Can you work these out from the model? Positions are in its coordinate system, mm. A direction names the side the tool comes from. Coordinates: 2 decimals unless noted, no trailing zeros. Loops run counter-clockwise (first coordinate to the right, second up) from the corner with the lowest first, then second, coordinate; pieces in that order, holes last.
Autodesk Inventor part; units mm, degrees
ref_plane "YZ Plane" through (0, 0, 0) normal (1, 0, 0) x (0, 1, 0)
ref_plane "XZ Plane" through (0, 0, 0) normal (0, 1, 0) x (-1, 0, 0)
ref_plane "XY Plane" through (0, 0, 0) normal (0, 0, 1) x (1, 0, 0)
sketch "Skizze3" plane through (0, 0, 0) normal (0, 1, 0) x (-1, 0, 0)
  line L0 (15, 237) -> (0, 237)
  line L1 (0, 237) -> (0, 0)
  line L2 (0, 0) -> (15, 0)
  line L3 (15, 0) -> (15, 237)
  line L4 (5, 134.5) -> (0, 134.5)
  line L5 (0, 134.5) -> (0, 102.5)
  line L6 (0, 102.5) -> (5, 102.5)
  line L7 (5, 102.5) -> (5, 134.5)
  point P0 (0, 134.5)
  dimension "d17" = 237
  dimension "d18" = 15
  dimension "d19" = 5
  dimension "d20" = 32
  dimension "d69" = 102.5
extrude "Extrusion4" add sketch "Skizze3" along normal blind 15 contours L3 L2 L1 L6 L7 L4 L0
sketch "Skizze6" plane through (0, 0, 0) normal (0, -1, 0) x (1, 0, 0)
  line L0 (0, 70) -> (-5, 0)
  line L1 (0, 0) -> (-15, 0)
  line L2 (0, 102.5) -> (0, 0)
  line L3 (-5, 237) -> (0, 167)
  line L4 (-15, 237) -> (0, 237)
  line L5 (0, 237) -> (0, 134.5)
  point P0 (0, 167)
  dimension "d48" = 0
  dimension "d49" = 10
  dimension "d50" = 0
  dimension "d51" = 70
  dimension "d52" = 0
  dimension "d53" = 10
  dimension "d54" = 70
  dimension "d55" = 0
extrude "Extrusion9" cut sketch "Skizze6" against normal blind 20
sketch "Skizze9" plane through (-15, 0, 0) normal (-1, 0, 0) x (0, 0, 1)
  circle A0 centre (118.5, 7.5) radius 3.1
  line L0 (0, 0) -> (0, 15)
  line L1 (0, 15) -> (237, 15)
  dimension "d70" = 6.2
  dimension "d71" = 118.5
  dimension "d72" = 7.5
extrude "Extrusion12" cut sketch "Skizze9" against normal blind 10
sketch "Skizze10" plane through (-15, 0, 0) normal (-1, 0, 0) x (0, 0, 1)
  circle A0 centre (4.8, 7.5) radius 2.3
  line L0 (0, 15) -> (237, 15)
  circle A1 centre (159.74, 7.5) radius 2.3
  circle A2 centre (232.13, 7.5) radius 2.3
  circle A3 centre (27.66, 7.5) radius 2.3
  line L1 (0, 0) -> (0, 15)
  dimension "d80" = 4.6
  dimension "d84" = 7.5
  dimension "d85" = 4.6
  dimension "d86" = 4.6
  dimension "d87" = 4.6
  dimension "d88" = 227.33
  dimension "d89" = 4.8
  dimension "d90" = 7.5
  dimension "d91" = 22.86
  dimension "d92" = 7.5
  dimension "d93" = 154.94
  dimension "d94" = 7.5
sketch "Skizze11" plane through (-15, 0, 0) normal (-1, 0, 0) x (0, 0, 1)
  circle A0 centre (118.5, 7.5) radius 3.1
  circle A1 centre (118.5, 7.5) radius 6
  point P0 (0, 0)
  dimension "d81" = 12
extrude "Extrusion15" cut sketch "Skizze11" against normal blind 5
extrude "Extrusion16" cut sketch "Skizze10" against normal blind 8
sketch "Skizze12" plane through (-15, 0, 0) normal (-1, 0, 0) x (0, 0, 1)
  circle A0 centre (159.74, 7.5) radius 2.3
  circle A1 centre (232.13, 7.5) radius 2.3
  circle A2 centre (27.66, 7.5) radius 2.3
  circle A3 centre (4.8, 7.5) radius 2.3
  circle A4 centre (232.13, 7.5) radius 2.3
  circle A5 centre (232.13, 7.5) radius 3.5
  circle A6 centre (159.74, 7.5) radius 2.3
  circle A7 centre (159.74, 7.5) radius 3.5
  circle A8 centre (27.66, 7.5) radius 3.5
  circle A9 centre (4.8, 7.5) radius 3.5
  point P0 (0, 0)
  dimension "d97" = 7
  dimension "d98" = 7
  dimension "d99" = 7
  dimension "d100" = 7
extrude "Extrusion17" add sketch "Skizze12" along normal blind 3
chamfer "Fase3" distance 1.5 angle 45 4 edges at (-15, 7.5, 228.63) (-15, 7.5, 156.24) (-15, 7.5, 24.16) (-15, 7.5, 1.3)
properties part number "atx_mount"
Item 1: Suppose I cut it at B-B, the plane z = 159.74. Please give me the cut outline in (x, y), plus the area to 3 significant figures.
Results are:
outline: (-18, 4) - (-16.5, 4) - (-15, 2.5) - (-15, 0) - (0, 0) - (0, 15) - (-15, 15) - (-15, 12.5) - (-16.5, 11) - (-18, 11) - (-18, 9.8) - (-7, 9.8) - (-7, 5.2) - (-18, 5.2) - close
area: 198 mm2
Item 2: Suppose I cut it at C-C, the plane z = 27.66. Please give me the cut outline in (x, y).
Results are:
outline: (-18, 4) - (-16.5, 4) - (-15, 2.5) - (-15, 0) - (-3.02, 0) - (-3.02, 15) - (-15, 15) - (-15, 12.5) - (-16.5, 11) - (-18, 11) - (-18, 9.8) - (-7, 9.8) - (-7, 5.2) - (-18, 5.2) - close
Item 3: I need wall thicknesses on line 1 along Y through (x, z) = (-9.75, 159.74); line 2 along Z through (x, y) = (-16, 10.25); line 3 along Y through (x, z) = (-6, 118.5). Which ranges of each line are inside material? Lowest first, please.
Results are:
line 1: y = 0 to 5.2, 9.8 to 15
line 2: z = 1.9 to 7.7, 24.76 to 30.56, 156.84 to 162.64, 229.23 to 235.03
line 3: y = 0 to 4.4, 10.6 to 15
Item 4: We'd pull the mould along Y, two halves only. Please class faces 4 (the face through (-3, 7, 134.5)), 5 (the face through (-7, 8, 28)), 6 (the face through (-17.24, 10.917, 4.041)): +Y half, -Y half, draft (parallel to the pull), parting line (faces both ways), or undercut.
Results are:
face 4: draft
face 5: undercut
face 6: parting line
Item 5: I'm going to push flat-ended pins straight in: P1, Ø6, axis at y = 10.5, z = 118, coming from the -X side; P2, Ø7.5, axis at y = 8, z = 111.5, coming from the +X side; P3, Ø4, axis at y = 7.5, z = 4.8, coming from the -X side. Where does each tip first touch, or does it pass through?
Results are:
P1: stops at x = -15
P2: stops at x = -5
P3: stops at x = -7
Item 6: Suppose I cut it at A-A, the plane z = 118.5. Please give me the cut outline in (x, y), plus the area to 3 significant figures.
Results are:
outline: (-15, 0) - (-5, 0) - (-5, 4.4) - (-10, 4.4) - (-10, 1.5) - (-15, 1.5) - close; (-15, 13.5) - (-10, 13.5) - (-10, 10.6) - (-5, 10.6) - (-5, 15) - (-15, 15) - close
area: 59.0 mm2
Item 7: Suppose I cut it at D-D, the plane z = 193. Please give me the cut outline in (x, y), plus the area to 3 significant figures.
Results are:
outline: (-15, 0) - (-1.86, 0) - (-1.86, 15) - (-15, 15) - close
area: 197 mm2
Item 8: On a 3-axis mill with a long thin cutter (end or side, diameter ignored), from which of +Z, -Z, +X, -X, +Y, -Y can I reach the whole of each face in a straight line? I mean faces 1 (the face through (-5, 4, 118)), 2 (the face through (-10, 7, 237)), 3 (the face through (-12.423, 8.381, 161.865)). Say none if no direction works.
Results are:
face 1: +X, +Y, -Y
face 2: +Z, +X, -X, +Y, -Y
face 3: -X
